Can you work these out from the model? Positions are in its coordinate system, mm. A direction names the side the tool comes from. Coordinates: 2 decimals unless noted, no trailing zeros. Order: outer loops, then holes, each group sorted by start corner. A loop starts at its lowest first (then second) coordinate and runs counter-clockwise, first axis right, second up.
```python
from build123d import *

# Parameters (mm, degrees)
ESQUISSE1_R        = 10.125
ESQUISSE1_R_2      = 8.125
BOSS_EXTRU_1_DEPTH = 4.5
ESQUISSE1_3_R      = 1.75
BOSS_EXTRU_2_DEPTH = 2
CONG_1_R           = 3.5
CONG_2_R           = 10


with BuildPart() as part:
    # Esquisse1 → Boss.-Extru.1 (new body)
    with BuildSketch(Plane.XY):
        Circle(ESQUISSE1_R)
        Circle(ESQUISSE1_R_2, mode=Mode.SUBTRACT)
    extrude(amount=BOSS_EXTRU_1_DEPTH)

    # Esquisse1<3> → Boss.-Extru.2 (add)
    with BuildSketch(Plane.XY):
        with BuildLine():
            Line((-15.028017241, 21.875), (-10.125, 0))
            ThreePointArc((-10.125, 0), (0, 10.125), (10.125, 0))
            Line((10.125, 0), (15.028017241, 21.875))
            Line((15.028017241, 21.875), (-15.028017241, 21.875))
        make_face()
        with Locations((-10.4375, 18.125)):
            Circle(ESQUISSE1_3_R, mode=Mode.SUBTRACT)
        with Locations((10.4375, 18.125)):
            Circle(ESQUISSE1_3_R, mode=Mode.SUBTRACT)
    extrude(amount=BOSS_EXTRU_2_DEPTH)

    # Congé1
    cong_1_edges = [part.edges().sort_by_distance(p)[0] for p in [
        (15.028017241, 21.875, 1),
        (-15.028017241, 21.875, 1),
    ]]
    fillet(cong_1_edges, radius=CONG_1_R)

    # Congé2
    # the kernel refuses this fillet: 10 mm, written as the material it adds along each edge
    with BuildSketch(Plane(origin=(-10.125, 0, 0), x_dir=(0.03212219246103637, -0.9994839492215452, 0), z_dir=(0, 0, 1))) as cong_2_piece_1:
        with BuildLine():
            CenterArc((0.971696322, -9.994839492), CONG_2_R, 91.840782713, 8.951796508)
            Line((-0.900844579, -0.171724377), (0, 0))
            ThreePointArc((0, 0), (0.325237199, -0.005225014), (0.650474397, 0))
        make_face()
    extrude(amount=2)
    with BuildSketch(Plane(origin=(10.125, 0, 0), x_dir=(0.21871145691738353, 0.9757895770160058, 0), z_dir=(0, 0, 1))) as cong_2_piece_2:
        with BuildLine():
            CenterArc((0.917066092, -10), CONG_2_R, 90, 8.951796508)
            ThreePointArc((-0.638968488, -0.121803991), (-0.318505839, -0.066034587), (0, 0))
            Line((0, 0), (0.917066092, 0))
        make_face()
    extrude(amount=2)


solid = part.part
```
1. Imagine slicing it at C-C on z = 3.4. Please give me the cut outline in (x, y) (3 decimals).
Completed:
outline: circle Ø20.25 at (0, 0); hole circle Ø16.25 at (0, 0)
2. Imagine slicing it at D-D on y = 9. Please give me the cut outline in (x, z), then the cut area to 3 significant figures.
Completed:
outline: (-12.14, 0) - (12.14, 0) - (12.14, 2) - (4.64, 2) - (4.64, 4.5) - (-4.64, 4.5) - (-4.64, 2) - (-12.14, 2) - close
area: 71.8 mm2
3. Imagine slicing it at B-B on y = 0. Please give me the cut outline in (x, z) (3 decimals).
Completed:
outline: (-10.167, 0) - (-8.125, 0) - (-8.125, 4.5) - (-10.125, 4.5) - (-10.125, 2) - (-10.167, 2) - close; (8.125, 0) - (10.167, 0) - (10.167, 2) - (10.125, 2) - (10.125, 4.5) - (8.125, 4.5) - close
4. Please list where these lines run through material, in increasing order: probe 1 along Y at (x, z) = (0, 1.4) (3 decimals); probe 2 along Y at (x, z) = (0, 2.75) (3 decimals); probe 3 along X at (y, z) = (19, 1.5).
Completed:
probe 1: y = -10.125 to -8.125, 8.125 to 21.875
probe 2: y = -10.125 to -8.125, 8.125 to 10.125
probe 3: x = -14.1 to -11.95, -8.92 to 8.92, 11.95 to 14.1
5. I'm going to push a flat-ended pin straight in: pin 1 (3 mm diameter, centred on x = 6.5, y = 10, fed in from +Z). Where does the tip first touch, or does it pass through?
Completed:
pin 1: stops at z = 2
6. Thinking about a two-plate mould opening in X: for faces 1 (the cylindrical face through (7.75, 2.44, 2.22)), 2 (the cylindrical face through (-13.416, 20.528, 1.014)), 3 (the cylindrical face through (10.21, 19.86, 0.99)), 4 (the flat face through (12.173, 9.135, 0.986)), which applies, pulls with the +X half, pulls with the -X half, needs draft (parallel to the pull), parting line crosses it, or undercut?
Completed:
face 1: undercut
face 2: pulls with the -X half
face 3: undercut
face 4: pulls with the +X half
7. Imagine slicing it at A-A on x = 0. Please give me the cut outline in (y, z) (3 decimals).
Completed:
outline: (-10.125, 0) - (-8.125, 0) - (-8.125, 4.5) - (-10.125, 4.5) - close; (8.125, 0) - (21.875, 0) - (21.875, 2) - (10.125, 2) - (10.125, 4.5) - (8.125, 4.5) - close
8. On a 3-axis mill with a long thin cutter (end or side, diameter ignored), from which of +Z, -Z, +X, -X, +Y, -Y can I reach the whole of each face in a straight line? I mean faces 5 (the cylindrical face through (4.672, -8.983, 2.718)), 6 (the flat face through (-12.225, 9.369, 0.986)). Say none if no direction works.
Completed:
face 5: +Z
face 6: +Z, -Z, -X, -Y
